Geometry: final body of the model. Coordinates: model frame, mm. A direction names the side the tool comes from. Coordinates: 2 decimals unless noted, no trailing zeros. Write each loop counter-clockwise with the first axis right and the second up, starting at its lowest first coordinate (ties: lowest second). Pieces come first, ordered by that corner, then holes. Notation, with made-up numbers: (71, 57.25) - (130, 57.25) arc R22 cw to (130, 89.25) - close; hole circle Ø9 at (2.5, 33). An arc over 180 degrees is marked (long way). Answer as a JSON object with one key per item and string values. Group by question number.
Item 1: First-contact query: pin 1 Ø6 at (x, y) = (9.5, 7) entering from -Z; pin 2 Ø0.9 at (x, y) = (11.5, 4.5) entering from +Z; pin 3 Ø1 at (x, z) = (10, -6) entering from -Y. Flat tips, straight axial feed; report the tip coordinate or a pass-through.
Item 2: Section B-B on y = 0. Return loops of the section in (x, z) (1 decimal).
Item 3: Section D-D on x = 4.5. Return loops of the section in (y, z), and give its area (3 significant figures).
Item 4: Line query: line 1 along Y through (x, z) = (12.9, 0); line 2 along Y through (x, z) = (14.1, 0); line 3 along X through (y, z) = (-6.5, 4.5). Output: solid intervals per line, ascending. Write a range as from..to.
Item 5: Section A-A on x = 12.5. Return loops of the section in (y, z).
Item 6: Mould query, pull axis Z, two halves, no side actions, for faces 1 (the flat face through (13.716, 2, -7)), 2 (the cylindrical face through (14.489, -10.074, -1.323)), 3 (the flat face through (12.4, 4.4, 0.991)). Classes: pulls with the +Z half, pulls with the -Z half, needs draft (parallel to the pull), parting line crosses it, or undercut.
Item 7: Set-up query: faces 4 (the cylindrical face through (7.33, 6.695, -1.487)), 5 (the flat face through (0, 0, 0)), 6 (the flat face through (12.4, 4.4, -0.991)). Return all of +Z, -Z, +X, -X, +Y, -Y with unobstructed straight access to the full face (end or side cutting, diameter ignored); none if empty.
```python
from build123d import *

# Parameters (mm, degrees)
CHAMFER1_SIZE  = 0.762
EXTRUDE1_DEPTH = 0.9906


with BuildPart() as part:
    # Sketch1 → Revolve1 (revolve)
    with BuildSketch(Plane.XY, mode=Mode.PRIVATE) as revolve1_sk:
        Polygon((0, 0), (0, 6.858), (13.716, 6.858), (13.716, 10.16), (15.24, 10.16), (15.24, 4.0005), (9.525, 4.0005), (9.525, 0), align=None)
    revolve(revolve1_sk.sketch.rotate(Axis((0, 0, 0), (1, 0, 0)), 90), axis=Axis((0, 0, 0), (1, 0, 0)))

    # Chamfer1
    chamfer1_edges = [part.edges().sort_by_distance(p)[0] for p in [
        (0, 0, -6.858),
    ]]
    chamfer(chamfer1_edges, length=CHAMFER1_SIZE)

    # Sketch3 → Extrude1 (cut, symmetric)
    with BuildSketch(Plane.XY):
        with BuildLine():
            Line((15.24, 4.9911), (11.519183101, 4.9911))
            ThreePointArc((11.519183101, 4.9911), (10.363552883, 4.677488096), (9.525, 3.8227))
            Line((9.525, 3.8227), (15.24, 3.8227))
            Line((15.24, 3.8227), (15.24, 4.9911))
        make_face()
    extrude(amount=EXTRUDE1_DEPTH, both=True, mode=Mode.SUBTRACT)


solid = part.part
```
Checks:
{
 "1": {"pin 1": "z = -5.57", "pin 2": "z = 5.53", "pin 3": "y = -4.1"},
 "2": {"outline": "(0, -6.1) - (0.8, -6.9) - (13.7, -6.9) - (13.7, -10.2) - (15.2, -10.2) - (15.2, -4) - (9.5, -4) - (9.5, 4) - (15.2, 4) - (15.2, 10.2) - (13.7, 10.2) - (13.7, 6.9) - (0.8, 6.9) - (0, 6.1) - close"},
 "3": {"outline": "circle Ø13.72 at (0, 0)", "area": "148 mm^2"},
 "4": {"line 1": "-6.86..-4, 4.99..6.86", "line 2": "-10.16..-4, 4.99..10.16", "line 3": "13.72..15.24"},
 "5": {"outline": "circle Ø13.72 at (0, 0); hole (3.88, -0.99) - (4.99, -0.99) - (4.99, 0.99) - (3.88, 0.99) arc R4 ccw (long way) to start"},
 "6": {"face 1": "needs draft", "face 2": "parting line crosses it", "face 3": "undercut"},
 "7": {"face 4": "-X", "face 5": "+Z, -Z, -X, +Y, -Y", "face 6": "+X"}
}
